For this review, take the finished solid that the model builds, in its own axes (mm). Give positions to 0.01 mm unless a question says otherwise; leave off trailing zeros. Write each loop counter-clockwise with the first axis right and the second up, starting at its lowest first coordinate (ties: lowest second). Pieces come first, ordered by that corner, then holes. Notation, with made-up numbers: (-18, 30.5) -> (11, 30.5) arc R16 cw to (11, 34.5) -> close; hole circle Ø6 at (62.5, -15.5). An arc over 180 degrees is marked (long way). Return JSON: item names as keys, results as strings.
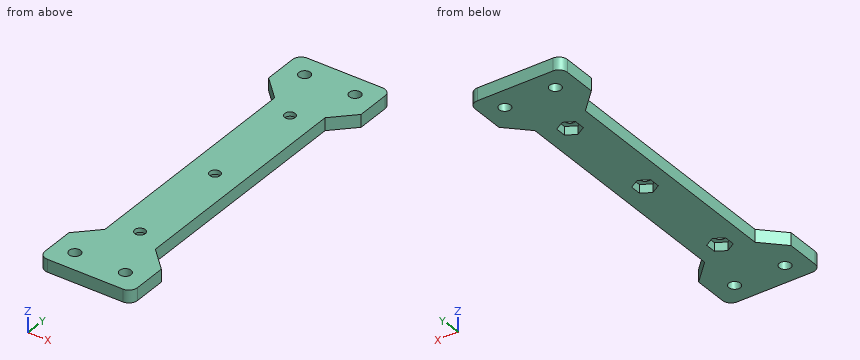
Autodesk Inventor part; units mm, degrees
ref_plane "YZ Plane" through (0, 0, 0) normal (1, 0, 0) x (0, 1, 0)
ref_plane "XZ Plane" through (0, 0, 0) normal (0, 1, 0) x (-1, 0, 0)
ref_plane "XY Plane" through (0, 0, 0) normal (0, 0, 1) x (1, 0, 0)
sketch "Sketch1" plane through (0, 0, 0) normal (0, 0, 1) x (1, 0, 0)
  line L0 (12.5, 0) -> (18.7, 0) construction
  line L1 (12.5, 0) -> (12.5, -92) construction
  line L2 (12.5, -92) -> (18.7, -92) construction
  line L3 (18.7, -90.35) -> (18.7, -92) construction
  line L4 (18.7, -90.35) -> (19, -90.0495) construction
  line L5 (19, -90.0495) -> (19, -83.1505) construction
  line L6 (19, -83.1505) -> (18.7, -82.85) construction
  line L7 (18.7, -13.75) -> (18.7, -82.85) construction
  line L8 (18.7, -13.75) -> (19, -13.4495) construction
  line L9 (19, -13.4495) -> (19, -6.5505) construction
  line L10 (19, -6.5505) -> (18.7, -6.25) construction
  line L11 (18.7, 0) -> (18.7, -6.25) construction
  circle A0 centre (16, -86.6) radius 1.25 construction
  circle A1 centre (16, -10) radius 1.25 construction
  line L12 (0.5, 0) -> (6.7, 0) construction
  line L13 (0.5, 0) -> (0.5, -92) construction
  line L14 (0.5, -92) -> (6.7, -92) construction
  line L15 (6.7, -90.35) -> (6.7, -92) construction
  line L16 (6.7, -90.35) -> (7, -90.0495) construction
  line L17 (7, -90.0495) -> (7, -83.1505) construction
  line L18 (7, -83.1505) -> (6.7, -82.85) construction
  line L19 (6.7, -13.75) -> (6.7, -82.85) construction
  line L20 (6.7, -13.75) -> (7, -13.4495) construction
  line L21 (7, -13.4495) -> (7, -6.5505) construction
  line L22 (7, -6.5505) -> (6.7, -6.25) construction
  line L23 (6.7, 0) -> (6.7, -6.25) construction
  circle A2 centre (4, -86.6) radius 1.25 construction
  circle A3 centre (4, -10) radius 1.25 construction
  circle A4 centre (4, -86.6) radius 1.375
  circle A5 centre (16, -86.6) radius 1.375
  circle A6 centre (16, -10) radius 1.375
  circle A7 centre (4, -10) radius 1.375
  line L24 (4, -86.6) -> (4, -10) construction
  line L25 (4, -10) -> (16, -10) construction
  line L26 (16, -10) -> (16, -86.6) construction
  line L27 (16, -86.6) -> (4, -86.6) construction
  line L28 (-1, -5) -> (-1, -91.6)
  line L29 (-1, -91.6) -> (21, -91.6)
  line L30 (21, -91.6) -> (21, -5)
  line L31 (21, -5) -> (-1, -5)
  point P0 (0, 0)
  dimension "d0" = 2.75
  dimension "d1" = 2.75
  dimension "d2" = 2.75
  dimension "d3" = 2.75
  dimension "d4" = 5
extrude "Extrusion1" add sketch "Sketch1" along normal blind 3
sketch "Sketch2" plane through (0, 0, 3) normal (0, 0, 1) x (1, 0, 0)
  line L0 (-1, -91.6) -> (21, -91.6)
  line L1 (21, -91.6) -> (21, -5)
  line L2 (21, -5) -> (-1, -5)
  line L3 (-1, -5) -> (-1, -91.6)
  circle A0 centre (4, -86.6) radius 1.375
  circle A1 centre (16, -86.6) radius 1.375
  circle A2 centre (16, -10) radius 1.375
  circle A3 centre (4, -10) radius 1.375
  line L4 (-1, -81.6) -> (4, -76.6)
  line L5 (4, -76.6) -> (4, -20)
  line L6 (4, -20) -> (-1, -15)
  point P0 (0, 0)
  dimension "d7" = 5
  dimension "d8" = 45
  dimension "d9" = 45
  dimension "d10" = 10
  dimension "d11" = 10
extrude "Extrusion2" cut sketch "Sketch2" against normal through all contours L3 L6 L5 L4
ref_plane "Work Plane1" through (10, -91.6, 0) normal (-1, 0, 0) x (0, 0, 1)
mirror "Mirror1" about plane through (10, -91.6, 0) normal (-1, 0, 0) of "Extrusion2"
sketch "Sketch3" plane through (0, 0, 3) normal (0, 0, 1) x (1, 0, 0)
  line L0 (16, -20) -> (21, -15)
  line L1 (21, -15) -> (21, -5)
  line L2 (21, -5) -> (-1, -5)
  line L3 (-1, -5) -> (-1, -15)
  line L4 (-1, -15) -> (4, -20)
  line L5 (4, -20) -> (4, -76.6)
  line L6 (4, -76.6) -> (-1, -81.6)
  line L7 (-1, -81.6) -> (-1, -91.6)
  line L8 (-1, -91.6) -> (21, -91.6)
  line L9 (21, -91.6) -> (21, -81.6)
  line L10 (21, -81.6) -> (16, -76.6)
  line L11 (16, -76.6) -> (16, -20)
  circle A0 centre (4, -86.6) radius 1.375
  circle A1 centre (16, -86.6) radius 1.375
  circle A2 centre (16, -10) radius 1.375
  circle A3 centre (4, -10) radius 1.375
  circle A4 centre (10, -48.3) radius 1.25
  line L12 (10, -91.6) -> (10, -48.3)
  line L13 (10, -48.3) -> (4, -48.3)
  point P0 (0, 0)
  dimension "d14" = 2.5
  dimension "d15" = 43.3
  dimension "d16" = 86.6
extrude "Extrusion3" cut sketch "Sketch3" against normal through all contours L12 L13 A4 | A4 L13 L12
sketch "Sketch4" plane through (0, 0, 0) normal (0, 0, -1) x (-1, 0, 0)
  circle A0 centre (-10, -48.3) radius 1.25
  line L0 (-10, -50.8981) -> (-12.25, -49.599)
  line L1 (-12.25, -49.599) -> (-12.25, -47.001)
  line L2 (-12.25, -47.001) -> (-10, -45.7019)
  line L3 (-10, -45.7019) -> (-7.75, -47.001)
  line L4 (-7.75, -47.001) -> (-7.75, -49.599)
  line L5 (-7.75, -49.599) -> (-10, -50.8981)
  line L6 (-4, -76.6) -> (-4, -20)
  point P0 (0, 0)
  dimension "d19" = 4.5
extrude "Extrusion4" cut sketch "Sketch4" against normal blind 2 contours A0 | L0 L1 L2 L3 L4 L5
pattern_linear "Rectangular Pattern1" count 3 spacing 25 along (0, -1, 0) of "Extrusion3", "Extrusion4" first direction both ways yes
ref_plane "Work Plane2" through (-1, -48.3, 0) normal (0, 1, 0) x (1, 0, 0)
fillet "Fillet1" radius 2 4 edges at (-1, -91.6, 1.5) (21, -91.6, 1.5) (-1, -5, 1.5) (21, -5, 1.5)
equation "\"d1\" = d0"
equation "\"d2\" = d0"
equation "\"d3\" = d0"
equation "\"d9\" = d8"
equation "\"d11\" = d10"
equation "\"d15\" = 0.5 * d16"
properties part number "A-06"
1. For pin 1 (0.6 mm diameter, centred on y = -48, z = 1, fed in from +X); pin 2 (2.5 mm diameter, centred on x = 9.5, y = -48, fed in from -Z); pin 3 (1.5 mm diameter, centred on y = -41.5, z = 2, fed in from -X); pin 4 (4.5 mm diameter, centred on x = 4, y = -10, fed in from -Z), all flat-tipped, find the tip position at first contact; note any pin that passes through.
Results found:
{"pin 1": "stops at x = 16", "pin 2": "stops at z = 2", "pin 3": "stops at x = 4", "pin 4": "stops at z = 0"}
2. Add section B-B, the plane y = -86.6. State the section outline as (x, z) points (3 decimals), plus the area to 3 significant figures.
Results found:
{"outline": "(-1, 0) -> (2.625, 0) -> (2.625, 3) -> (-1, 3) -> close; (5.375, 0) -> (14.625, 0) -> (14.625, 3) -> (5.375, 3) -> close; (17.375, 0) -> (21, 0) -> (21, 3) -> (17.375, 3) -> close", "area": "49.5 mm²"}
3. Add section D-D, the plane y = -58. State the section outline as (x, z) points.
Results found:
{"outline": "(4, 0) -> (16, 0) -> (16, 3) -> (4, 3) -> close"}
4. To check wall thickness, follow probe 1 along Y at (x, z) = (10, 2.7); probe 2 along X at (y, z) = (-86.6, 1.05) (3 decimals); probe 3 along Y at (x, z) = (5, 0.3). State the ranges of each line that lie inside material, in increasing order.
Results found:
{"probe 1": "y = -91.6 to -74.55, -72.05 to -49.55, -47.05 to -24.55, -22.05 to -5", "probe 2": "x = -1 to 2.625, 5.375 to 14.625, 17.375 to 21", "probe 3": "y = -91.6 to -87.54, -85.66 to -10.94, -9.06 to -5"}
5. Add section C-C, the plane z = 1.55. Count the separate pieces of the cut face and the enclosed holes in it, plus the area to 3 significant figures.
Results found:
{"separate pieces": "1", "enclosed holes": "7", "area": "1,210 mm²"}
6. Add section A-A, the plane y = -48.3. State the section outline as (x, z) points.
Results found:
{"outline": "(4, 0) -> (7.75, 0) -> (7.75, 2) -> (8.75, 2) -> (8.75, 3) -> (4, 3) -> close; (11.25, 2) -> (12.25, 2) -> (12.25, 0) -> (16, 0) -> (16, 3) -> (11.25, 3) -> close"}
